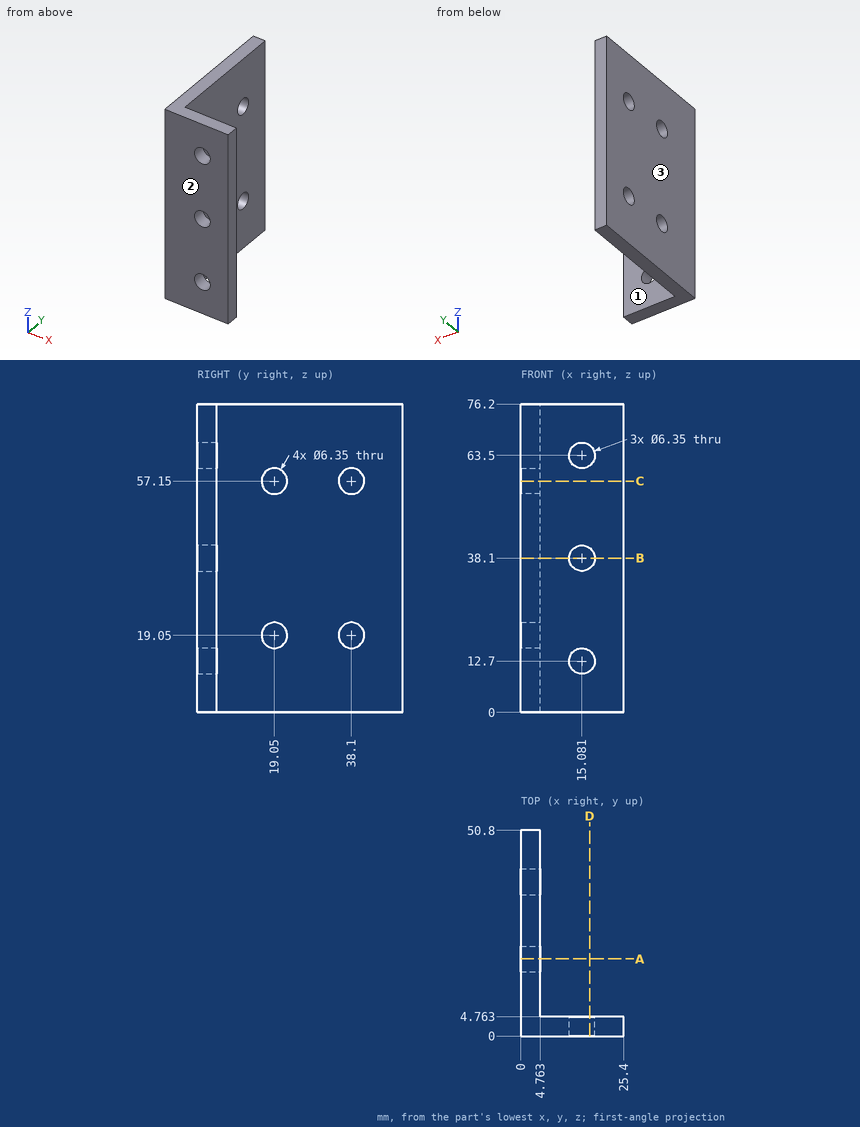
Print and shaded views of the part. All mm, measured from the part's lowest x, y and z. Give positions to 0.01 mm unless a question says otherwise; leave off trailing zeros. Write each loop counter-clockwise with the first axis right and the second up, starting at its lowest first coordinate (ties: lowest second). Pieces come first, ordered by that corner, then holes. Notation, with made-up numbers: (80, 34) - (85, 34) arc R22 ccw to (85, 60) - close; hole circle Ø11 at (-22.75, -38). An arc over 180 degrees is marked (long way). One line per question, with ' | ' between items. Start each with the question number.
(1) Slice it at B-B on z = 38.1. Write the cut outline in (x, y).
(2) Pin check, flat tip, straight feed: P1, Ø7.5, axis at y = 19.05, z = 57.15, coming from the +X side. Stop position of the tip, or through.
(3) Two-plate mould, pull along Y, no slides. Class the marked faces 1, 2 and 3: +Y half, -Y half, draft (parallel to the pull), parting line (faces both ways), or undercut.
(4) Slice it at A-A on y = 19.05. Write the cut outline in (x, z) (1 decimal).
(5) Slice it at D-D on x = 17. Write the cut outline in (y, z).
(6) Slice it at C-C on z = 57.15. Write the cut outline in (x, y) (1 decimal), plus the area to 3 significant figures.
(7) Wall check: line 1 along Y through (x, z) = (3.25, 57.15) (1 decimal); line 2 along X through (y, z) = (3.7, 63.5); line 3 along X through (y, z) = (6.5, 50). Give the ranges that are in metal, low to high. Write a range as from..to.
Results below:
1) outline: (0, 0) - (11.91, 0) - (11.91, 4.76) - (4.76, 4.76) - (4.76, 50.8) - (0, 50.8) - close; (18.26, 0) - (25.4, 0) - (25.4, 4.76) - (18.26, 4.76) - close
2) P1: x = 4.76
3) face 1: +Y half | face 2: -Y half | face 3: draft
4) outline: (0, 0) - (4.8, 0) - (4.8, 15.9) - (0, 15.9) - close; (0, 22.2) - (4.8, 22.2) - (4.8, 54) - (0, 54) - close; (0, 60.3) - (4.8, 60.3) - (4.8, 76.2) - (0, 76.2) - close
5) outline: (0, 0) - (4.76, 0) - (4.76, 10.17) - (0, 10.17) - close; (0, 15.23) - (4.76, 15.23) - (4.76, 35.57) - (0, 35.57) - close; (0, 40.63) - (4.76, 40.63) - (4.76, 60.97) - (0, 60.97) - close; (0, 66.03) - (4.76, 66.03) - (4.76, 76.2) - (0, 76.2) - close
6) outline: (0, 0) - (25.4, 0) - (25.4, 4.8) - (4.8, 4.8) - (4.8, 15.9) - (0, 15.9) - close; (0, 22.2) - (4.8, 22.2) - (4.8, 34.9) - (0, 34.9) - close; (0, 41.3) - (4.8, 41.3) - (4.8, 50.8) - (0, 50.8) - close | area: 280 mm^2
7) line 1: 0..15.9, 22.2..34.9, 41.3..50.8 | line 2: 0..11.91, 18.26..25.4 | line 3: 0..4.76
